Part model, mm, in its own coordinate system. Face numbers are marked on the shaded views. A direction names the side the tool comes from. Coordinates: 2 decimals unless noted, no trailing zeros. Loops run counter-clockwise (first coordinate to the right, second up) from the corner with the lowest first, then second, coordinate; pieces in that order, holes last. Notation, with made-up numbers: M 73,-34 L 129,-34 A27 cw 129,-1 Z; hole C 8,-37 d9. An arc over 180 degrees is marked long. Answer as a JSON object with one key per item and string values. Group by question number.
1. Saw through at A-A on z = -84. Write the cut outline in (x, y).
2. Saw through at D-D on y = 55. Count the separate pieces of the cut face and the enclosed holes in it, then the cut area to 3 significant figures.
3. 3-axis set-ups, long thin cutter, end or side, ignore diameter. For the marked faces 1, 2, 3 and 4: which of +Z, -Z, +X, -X, +Y, -Y reach the whole face in a straight line?
4. Drill centre lines: L1, parallel to Z at x = 99, y = 13; L2, parallel to Z at x = 151.5, y = 66.5; L3, parallel to X at y = 67, z = -21.5. Where is each one in solid material? Low to high.
5. Mould opens along Z. For the marked faces 5, 6, 7 and 8 say: released by +Z, released by -Z, zero draft, split by the parting line, or undercut.
6. Saw through at C-C on y = 94. Write the cut outline in (x, z).
7. Drop flat-ended pins along their axis: pin 1 Ø12 at (x, y) = (88, 33.5) entering from -Z; pin 2 Ø18.5 at (x, y) = (18, 40) entering from -Z; pin 3 Ø12.5 at (x, y) = (59.04, 100.96) entering from +Z; pin 4 Ø4.5 at (x, z) = (25, -6) entering from -Y. Give the stop position or say it passes through.
8. Saw through at B-B on x = 139. Write the cut outline in (y, z), then the cut area to 3 significant figures.
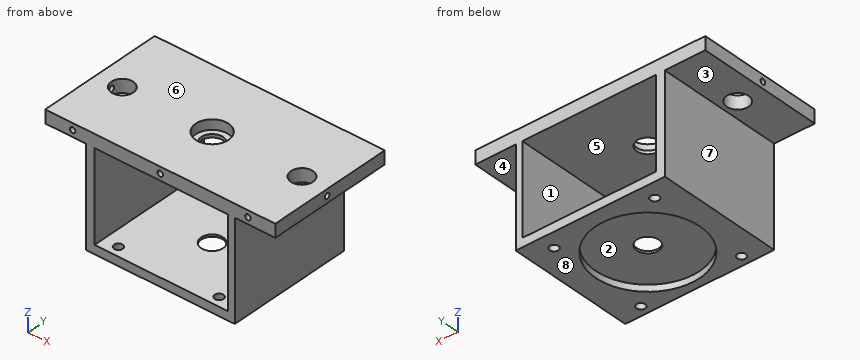
from build123d import *

# Parameters (mm, degrees)
SKETCH1_W                 = 210
SKETCH1_H                 = 12
BOSS_EXTRUDE1_DEPTH       = 116
SKETCH2_R                 = 10
CUT_EXTRUDE1_DEPTH        = 13
F_5_0MM_DOWEL_HOLE1_D     = 5
F_5_0MM_DOWEL_HOLE1_DEPTH = 25
F_5_0MM_DOWEL_HOLE1_TIP   = 1.502151548
F_5_0MM_DOWEL_HOLE2_D     = 5
F_5_0MM_DOWEL_HOLE2_DEPTH = 25
F_5_0MM_DOWEL_HOLE2_TIP   = 1.502151548
F_5_0MM_DOWEL_HOLE3_D     = 5
F_5_0MM_DOWEL_HOLE3_DEPTH = 25
F_5_0MM_DOWEL_HOLE3_TIP   = 1.502151548
SKETCH11_W                = 8
SKETCH11_H                = 116
SKETCH11_W_2              = 6
BOSS_EXTRUDE2_DEPTH       = 90
BOSS_EXTRUDE4_REACH       = 169
SKETCH12_W                = 8
SKETCH12_H                = 116
SKETCH7_R                 = 10
CUT_EXTRUDE3_DEPTH        = 103
SKETCH13_R                = 47.5
CUT_EXTRUDE4_DEPTH        = 6
CIRPATTERN1_COUNT         = 4
SKETCH16_R                = 15
CUT_EXTRUDE5_DEPTH        = 9


with BuildPart() as part:
    # Sketch1 → Boss-Extrude1 (new body)
    with BuildSketch(Plane(origin=(0, 0, 0), x_dir=(1, 0, 0), z_dir=(0, 1, 0))):
        with Locations((105, 6)):
            Rectangle(SKETCH1_W, SKETCH1_H)
    extrude(amount=BOSS_EXTRUDE1_DEPTH)

    # Sketch2 → Cut-Extrude1 (cut, through all)
    with BuildSketch(Plane.XY):
        with Locations((23, 55)):
            Circle(SKETCH2_R)
        with Locations((187, 55)):
            Circle(SKETCH2_R)
    extrude(amount=-CUT_EXTRUDE1_DEPTH, mode=Mode.SUBTRACT)

    # 5.0mm Dowel Hole1
    with Locations(Plane.ZY):
        with Locations((-6, 55)):
            Hole(F_5_0MM_DOWEL_HOLE1_D / 2, depth=F_5_0MM_DOWEL_HOLE1_DEPTH)
            with Locations((0, 0, -(F_5_0MM_DOWEL_HOLE1_DEPTH + F_5_0MM_DOWEL_HOLE1_TIP / 2))):  # 118° drill point
                Cone(0, F_5_0MM_DOWEL_HOLE1_D / 2, F_5_0MM_DOWEL_HOLE1_TIP, mode=Mode.SUBTRACT)

    # 5.0mm Dowel Hole2
    with Locations(Plane(origin=(210, 0, 0), x_dir=(0, 0, -1), z_dir=(1, 0, 0))):
        with Locations((6, 55)):
            Hole(F_5_0MM_DOWEL_HOLE2_D / 2, depth=F_5_0MM_DOWEL_HOLE2_DEPTH)
            with Locations((0, 0, -(F_5_0MM_DOWEL_HOLE2_DEPTH + F_5_0MM_DOWEL_HOLE2_TIP / 2))):  # 118° drill point
                Cone(0, F_5_0MM_DOWEL_HOLE2_D / 2, F_5_0MM_DOWEL_HOLE2_TIP, mode=Mode.SUBTRACT)

    # 5.0mm Dowel Hole3
    with Locations(Plane(origin=(0, 0, 0), x_dir=(-1, 0, 0), z_dir=(0, -1, 0))):
        with Locations((-25, 6), (-105, 6), (-185, 6)):
            Hole(F_5_0MM_DOWEL_HOLE3_D / 2, depth=F_5_0MM_DOWEL_HOLE3_DEPTH)
            with Locations((0, 0, -(F_5_0MM_DOWEL_HOLE3_DEPTH + F_5_0MM_DOWEL_HOLE3_TIP / 2))):  # 118° drill point
                Cone(0, F_5_0MM_DOWEL_HOLE3_D / 2, F_5_0MM_DOWEL_HOLE3_TIP, mode=Mode.SUBTRACT)

    # Sketch11 → Boss-Extrude2 (add)
    with BuildSketch(Plane(origin=(0, 0, -12), x_dir=(-1, 0, 0), z_dir=(0, 0, -1))):
        with Locations((-41, 58)):
            Rectangle(SKETCH11_W, SKETCH11_H)
        with Locations((-170, 58)):
            Rectangle(SKETCH11_W_2, SKETCH11_H)
    extrude(amount=BOSS_EXTRUDE2_DEPTH)

    # Sketch12 → Boss-Extrude4 (add, up to next)
    with BuildSketch(Plane.ZY.offset(-167), mode=Mode.PRIVATE) as boss_extrude4_sk1:
        with Locations((-98, 58)):
            Rectangle(SKETCH12_W, SKETCH12_H)
    boss_extrude4_tool1 = extrude(boss_extrude4_sk1.sketch, amount=BOSS_EXTRUDE4_REACH, mode=Mode.PRIVATE) - part.part
    add(boss_extrude4_tool1.solids().sort_by_distance((167, 58, -98))[0])

    # Sketch7 → Cut-Extrude3 (cut, through all)
    with BuildSketch(Plane.XY):
        with Locations((105, 55)):
            Circle(SKETCH7_R)
    extrude(amount=-CUT_EXTRUDE3_DEPTH, mode=Mode.SUBTRACT)

    # Sketch13 → Cut-Extrude4 (cut)
    with BuildSketch(Plane(origin=(0, 0, -102), x_dir=(-1, 0, 0), z_dir=(0, 0, -1))):
        with Locations((-105, 55)):
            Circle(SKETCH13_R)
    extrude(amount=-CUT_EXTRUDE4_DEPTH, mode=Mode.SUBTRACT)

    # Sketch14 → 5_16 _0.3125_ Diameter Hole1 (revolve, cut)
    with BuildSketch(Plane(origin=(150.961940777, 100.961940777, -102), x_dir=(0, 1, 0), z_dir=(1, 0, 0))):
        Polygon((0, 0), (0, 14.384665582), (3.96875, 12), (3.96875, 0), align=None)
    f_5_16_0_3125_diameter_hole1 = revolve(axis=Axis((150.961940777, 100.961940777, -108.35), (0, 0, 1)), mode=Mode.SUBTRACT)

    # CirPattern1: 5_16 _0.3125_ Diameter Hole1 ×4 about axis
    cirpattern1_axis = Axis((105, 55, 0), (0, 0, 1))
    for i in range(1, CIRPATTERN1_COUNT):
        add(f_5_16_0_3125_diameter_hole1.rotate(cirpattern1_axis, i * 360 / CIRPATTERN1_COUNT), mode=Mode.SUBTRACT)

    # Sketch16 → Cut-Extrude5 (cut)
    with BuildSketch(Plane.XY):
        with Locations((105, 55)):
            Circle(SKETCH16_R)
    extrude(amount=-CUT_EXTRUDE5_DEPTH, mode=Mode.SUBTRACT)


solid = part.part
Outcome:
{
 "1": {"outline": "M 37,0 L 45,0 L 45,116 L 37,116 Z; M 167,0 L 173,0 L 173,116 L 167,116 Z"},
 "2": {"separate pieces": "6", "enclosed holes": "0", "area": "3,210 mm²"},
 "3": {"face 1": "+Y, -Y", "face 2": "-Z", "face 3": "-Z, -X, +Y, -Y", "face 4": "-Z, +X, +Y, -Y"},
 "4": {"L1": "z = -96 to -94, -12 to 0", "L2": "z = -102 to -94, -12 to 0", "L3": "x = 37 to 45, 167 to 173"},
 "5": {"face 5": "undercut", "face 6": "released by +Z", "face 7": "zero draft", "face 8": "released by -Z"},
 "6": {"outline": "M 0,-12 L 37,-12 L 37,-102 L 77.88,-102 L 77.88,-96 L 132.12,-96 L 132.12,-102 L 173,-102 L 173,-12 L 210,-12 L 210,0 L 0,0 Z; hole M 45,-94 L 167,-94 L 167,-12 L 45,-12 Z"},
 "7": {"pin 1": "stops at z = -96", "pin 2": "stops at z = -12", "pin 3": "stops at z = 0", "pin 4": "stops at y = 25.15"},
 "8": {"outline": "M 0,-102 L 21.83,-102 L 21.83,-96 L 88.17,-96 L 88.17,-102 L 116,-102 L 116,-94 L 0,-94 Z; M 0,-12 L 116,-12 L 116,0 L 0,0 Z", "area": "1,920 mm²"}
}
